Design review of the part built by this model. Coordinates are the model's own, in mm. A direction names the side the tool comes from. Coordinates: 2 decimals unless noted, no trailing zeros. Order: outer loops, then holes, each group sorted by start corner. A loop starts at its lowest first (then second) coordinate and runs counter-clockwise, first axis right, second up. Notation, with made-up numbers: (-40, 83.25) -> (6, 83.25) arc R14 cw to (6, 107.25) -> close; hole circle Ø4 at (-34, 12.5). An arc over 180 degrees is marked (long way). Use a Markdown table: item, result. Add a question column.
Q1. Add section B-B (y = -9). State the section outline as (x, z) points, then the cut area to 3 significant figures.
Q2. Add section D-D (z = 36). State the section outline as (x, y) points.
Q3. The part is to be moulded in two halves that separate along Y. For faces 1 (the face through (0.638, -25.986, 31.007)), 2 (the face through (-35.43, 26.4, 30.42)), 3 (the face through (0, 0, 2)), say which applies: pulls with the +Y half, pulls with the -Y half, needs draft (parallel to the pull), parting line crosses it, or undercut.
Q4. Machinability: for faces 4 (the face through (34, 0, 31)), 5 (the face through (-36, 0, 30)), which of the approach directions +Z, -Z, +X, -X, +Y, -Y give a long, thin tool a straight path to every point of the face, cutting with its end or side? Answer none if there is none.
Q5. Insertion check: pin 1 (4 mm diameter, centred on x = -0.5, y = -9.5, fed in from +Z). The pin has a flat end and moves straight along its axis. Give the tip position at first contact, or say it passes through.
Q6. Add section A-A (z = 12). State the section outline as (x, y) points.
Q7. Add section C-C (x = 0). State the section outline as (y, z) points.
Q8. Wall thickness on probe 1 along X at (y, z) = (4, 11); probe 2 along Y at (x, z) = (-32, 30.5); probe 3 along Z at (x, y) = (-10.5, 23.5): over which ranges is each line inside the solid? List them lowest first.
from build123d import *

# Parameters (mm, degrees)
F0_W     = 68
F0_H     = 50
F1_DEPTH = 2
F0_W_2   = 72
F0_H_2   = 54
F2_DEPTH = 60
F4_DEPTH = 25
F5_R     = 2


# Not quite as in the source:
# - a feature names something its author has since deleted; it is built from what else it names


with BuildPart() as f1:
    # F0 (on Top) → F1 (new body)
    with BuildSketch(Plane.XY):
        Rectangle(F0_W, F0_H)
    extrude(amount=F1_DEPTH)

    # F0 (on Top) → F2 (join)
    with BuildSketch(Plane.XY):
        Rectangle(F0_W_2, F0_H_2)
        Rectangle(F0_W, F0_H, mode=Mode.SUBTRACT)
    extrude(amount=F2_DEPTH)

    # F3 (on face) → F4 (cut)
    with BuildSketch(Plane(origin=(0, -25, 0), x_dir=(-1, 0, 0), z_dir=(0, 1, 0))):
        with BuildLine():
            Line((29, 60), (-29, 60))
            ThreePointArc((-29, 60), (0, 31), (29, 60))
        make_face()
    extrude(amount=-F4_DEPTH, mode=Mode.SUBTRACT)

    # F5
    f5_edges = [f1.edges().sort_by_distance(p)[0] for p in [
        (-36, 27, 30),
        (36, 27, 30),
        (-36, -27, 30),
        (36, -27, 30),
    ]]
    fillet(f5_edges, radius=F5_R)


solid = f1.part
Established:
| question | item | result |
|---|---|---|
| 1 | outline | (-36, 0) -> (36, 0) -> (36, 60) -> (34, 60) -> (34, 2) -> (-34, 2) -> (-34, 60) -> (-36, 60) -> close |
| 1 | area | 376 mm^2 |
| 2 | outline | (-36, -25) arc R2 ccw to (-34, -27) -> (-16.28, -27) -> (-16.28, -25) -> (-34, -25) -> (-34, 25) -> (34, 25) -> (34, -25) -> (16.28, -25) -> (16.28, -27) -> (34, -27) arc R2 ccw to (36, -25) -> (36, 25) arc R2 ccw to (34, 27) -> (-34, 27) arc R2 ccw to (-36, 25) -> close |
| 3 | face 1 | needs draft |
| 3 | face 2 | pulls with the +Y half |
| 3 | face 3 | undercut |
| 4 | face 4 | +Z |
| 4 | face 5 | +Z, -Z, -X, +Y, -Y |
| 5 | pin 1 | z = 2 |
| 6 | outline | (-36, -25) arc R2 ccw to (-34, -27) -> (34, -27) arc R2 ccw to (36, -25) -> (36, 25) arc R2 ccw to (34, 27) -> (-34, 27) arc R2 ccw to (-36, 25) -> close; hole (-34, -25) -> (34, -25) -> (34, 25) -> (-34, 25) -> close |
| 7 | outline | (-27, 0) -> (27, 0) -> (27, 60) -> (25, 60) -> (25, 2) -> (-25, 2) -> (-25, 31) -> (-27, 31) -> close |
| 8 | probe 1 | -36 to -34, 34 to 36 |
| 8 | probe 2 | -27 to -25, 25 to 27 |
| 8 | probe 3 | 0 to 2 |
